Work out the finished part from the listing and answer in its coordinate system (mm). Coordinates: 2 decimals unless noted, no trailing zeros. Loops run counter-clockwise (first coordinate to the right, second up) from the corner with the lowest first, then second, coordinate; pieces in that order, holes last. Notation, with made-up numbers: (67.5, 85) - (105.5, 85) arc R13 cw to (105.5, 95) - close; hole circle Ø10 at (-4, 75.25). An arc over 180 degrees is marked (long way). Write each question's results on one line, items separated by ' | '. Start each with the question number.
Item 1: Consider probe 1 along Z at (x, y) = (-48.5, -0.1); probe 2 along X at (y, z) = (-0.2, 10); probe 3 along X at (y, z) = (-0.4, -1). Determine where each line is inside the solid, lowest interval first. Write a range as [from, to].
Item 2: Section A-A, the plane z = -11.5 is taken. Write down the section's boundary in (x, y), plus the area to 3 significant figures.
Item 3: For a pull along Z with two mould halves and no side action, classify faces 1 (the face through (-51.4, -0.76, 14.45)), 2 (the face through (-36.03, -0.76, 2.57)), 3 (the face through (-1, -1.5, 0)) as +Z half, -Z half, draft (parallel to the pull), parting line (faces both ways), or undercut.
Item 4: Section C-C, the plane y = -0.6 is taken. Write down the section's boundary in (x, z), plus the area to 3 significant figures.
Item 5: Section B-B, the plane x = -39.37 is taken. Write down the section's boundary in (y, z).
from build123d import *

# Parameters (mm, degrees)
SKETCH_W            = 104.8
SKETCH_H            = 31
PAD_DEPTH           = 1.5
HOLE_D              = 3.4
HOLE_DEPTH          = 25
HOLE_CSINK_D        = 6.1
HOLE_CSINK_ANGLE    = 90
FILLET_R            = 3.5
SKETCH002_R         = 3.5
POCKET_DEPTH        = 1.501
LINEARPATTERN_COUNT = 2
LINEARPATTERN_PITCH = 80.01


with BuildPart() as part:
    # Sketch → Pad (new body)
    with BuildSketch(Plane.XZ):
        Rectangle(SKETCH_W, SKETCH_H)
    extrude(amount=PAD_DEPTH)

    # Hole
    with Locations(Plane.XZ.offset(1.5)):
        with Locations((-48.5, 11.5), (-48.5, -11.5), (48.5, -11.5), (48.5, 11.5)):
            CounterSinkHole(HOLE_D / 2, HOLE_CSINK_D / 2, depth=HOLE_DEPTH, counter_sink_angle=HOLE_CSINK_ANGLE)

    # Fillet
    fillet_edges = [part.edges().sort_by_distance(p)[0] for p in [
        (-52.4, -0.75, 15.5),
        (52.4, -0.75, 15.5),
    ]]
    fillet(fillet_edges, radius=FILLET_R)

    # Sketch002 (on Face5 of Fillet) → Pocket (cut, through all)
    with BuildSketch(Plane.XZ.offset(1.5)):
        with Locations((-39.37, 1.52)):
            Circle(SKETCH002_R)
    pocket = extrude(amount=-POCKET_DEPTH, mode=Mode.SUBTRACT)

    # LinearPattern: Pocket ×2
    with Locations(*[(i * LINEARPATTERN_PITCH, 0, 0) for i in range(1, LINEARPATTERN_COUNT)]):
        add(pocket, mode=Mode.SUBTRACT)


solid = part.part
Answer key:
1) probe 1: z = [-15.5, -13.2], [-9.8, 9.8], [13.2, 15.5] | probe 2: x = [-52.4, -49.4], [-47.6, 47.6], [49.4, 52.4] | probe 3: x = [-52.4, -41.8], [-36.94, 38.21], [43.07, 52.4]
2) outline: (-52.4, -1.5) - (-51.55, -1.5) - (-50.2, -0.15) - (-50.2, 0) - (-52.4, 0) - close; (-46.8, -0.15) - (-45.45, -1.5) - (45.45, -1.5) - (46.8, -0.15) - (46.8, 0) - (-46.8, 0) - close; (50.2, -0.15) - (51.55, -1.5) - (52.4, -1.5) - (52.4, 0) - (50.2, 0) - close | area: 143 mm^2
3) face 1: +Z half | face 2: undercut | face 3: draft
4) outline: (-52.4, -15.5) - (52.4, -15.5) - (52.4, 12) arc R3.5 ccw to (48.9, 15.5) - (-48.9, 15.5) arc R3.5 ccw to (-52.4, 12) - close; hole circle Ø4.3 at (-48.5, -11.5); hole circle Ø4.3 at (-48.5, 11.5); hole circle Ø7 at (-39.37, 1.52); hole circle Ø7 at (40.64, 1.52); hole circle Ø4.3 at (48.5, -11.5); hole circle Ø4.3 at (48.5, 11.5) | area: 3,110 mm^2
5) outline: (-1.5, -15.5) - (0, -15.5) - (0, -1.98) - (-1.5, -1.98) - close; (-1.5, 5.02) - (0, 5.02) - (0, 15.5) - (-1.5, 15.5) - close
